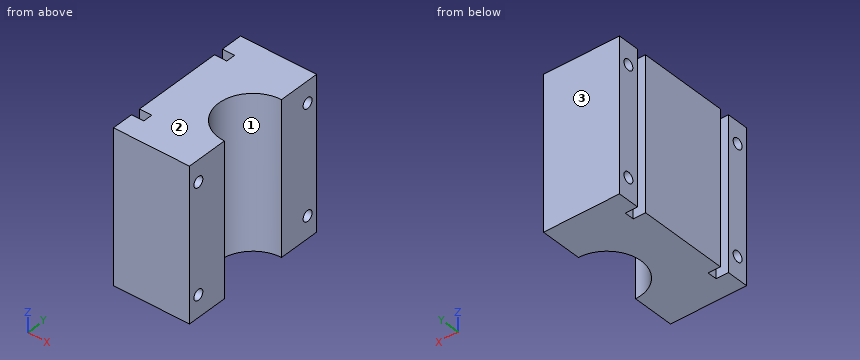
from build123d import *

# Parameters (mm, degrees)
F1_DEPTH = 50.8
F2_DEPTH = 50.8
F4_D     = 7.112


with BuildPart() as f1:
    # F0 (on Top) → F1 (new body)
    with BuildSketch(Plane.XY):
        with BuildLine():
            Line((-50.8, 0), (-22.86, 0))
            ThreePointArc((-22.86, 0), (-16.164461, 16.164461), (0, 22.86))
            Line((0, 22.86), (0, 50.8))
            Line((0, 50.8), (-50.8, 50.8))
            Line((-50.8, 50.8), (-50.8, 36.323187))
            Line((-50.8, 36.323187), (-42.600878, 36.323187))
            Line((-42.600878, 36.323187), (-42.600878, 29.973187))
            Line((-42.600878, 29.973187), (-50.8, 29.973187))
            Line((-50.8, 29.973187), (-50.8, 0))
        make_face()
        with BuildLine():
            ThreePointArc((0, -22.86), (-16.164461, -16.164461), (-22.86, 0))
            Line((-22.86, 0), (-50.8, 0))
            Line((-50.8, 0), (-50.8, -29.973187))
            Line((-50.8, -29.973187), (-42.600878, -29.973187))
            Line((-42.600878, -29.973187), (-42.600878, -36.323187))
            Line((-42.600878, -36.323187), (-50.8, -36.323187))
            Line((-50.8, -36.323187), (-50.8, -50.8))
            Line((-50.8, -50.8), (0, -50.8))
            Line((0, -50.8), (0, -22.86))
        make_face()
    extrude(amount=F1_DEPTH)

    # F1_face (on face) → F2 (join)
    with BuildSketch(Plane(origin=(-27.91822, 0, 50.8), x_dir=(1, 0, 0), z_dir=(0, 0, 1))):
        with BuildLine():
            Line((-14.682658, 36.323187), (-14.682658, 29.973187))
            Line((-14.682658, 29.973187), (-22.88178, 29.973187))
            Line((-22.88178, 29.973187), (-22.88178, -29.973187))
            Line((-22.88178, -29.973187), (-14.682658, -29.973187))
            Line((-14.682658, -29.973187), (-14.682658, -36.323187))
            Line((-14.682658, -36.323187), (-22.88178, -36.323187))
            Line((-22.88178, -36.323187), (-22.88178, -50.8))
            Line((-22.88178, -50.8), (27.91822, -50.8))
            Line((27.91822, -50.8), (27.91822, -22.86))
            ThreePointArc((27.91822, -22.86), (5.05822, 0), (27.91822, 22.86))
            Line((27.91822, 22.86), (27.91822, 50.8))
            Line((27.91822, 50.8), (-22.88178, 50.8))
            Line((-22.88178, 50.8), (-22.88178, 36.323187))
            Line((-22.88178, 36.323187), (-14.682658, 36.323187))
        make_face()
    extrude(amount=F2_DEPTH)

    # F4 (through all)
    with Locations(Plane(origin=(-50.8, 0, 0), x_dir=(0, -1, 0), z_dir=(-1, 0, 0))):
        with Locations((-43.662325, 87.244935), (43.662325, 87.244935), (43.662325, 14.645034), (-43.662325, 14.645034)):
            Hole(F4_D / 2)


solid = f1.part
Input: part model. Units: mm. Frame: model coordinates. Face numbers are marked on the shaded views. Coordinates: 2 decimals unless noted, no trailing zeros. Loops run counter-clockwise (first coordinate to the right, second up) from the corner with the lowest first, then second, coordinate; pieces in that order, holes last.
Q1. Cut plane B-B (z = 89). Output: boundary loops of the cut face in (x, y), then the cut area to 3 significant figures.
Q2. Contact query for flat-ended pins moving along their axis: pin 1 (11.5 mm diameter, centred on y = 43.66, z = 87.24, fed in from +X); pin 2 (3 mm diameter, centred on y = 34, z = 44, fed in from -X); pin 3 (5.5 mm diameter, centred on y = 43.66, z = 14.65, fed in from +X). Output: stop coordinate, or through.
Q3. Cut plane A-A (x = -20). Output: boundary loops of the cut face in (y, z).
Q4. Draft query along Y for the marked faces 1, 2 and 3. Return one class per face: +Y half, -Y half, draft (parallel to the pull), parting line (faces both ways), or undercut.
Q5. Material intervals for line 1 (Z direction, x = -23, y = -44) (3 decimals); line 2 (Z direction, x = -46, y = -45); line 3 (Y direction, x = -14, z = 87), sorted ascending.
Q6. Cut plane C-C (x = -46.5). Output: boundary loops of the cut face in (y, z), then the cut area to 3 significant figures.
Q7. Cut plane D-D (z = 41). Output: boundary loops of the cut face in (x, y).
Working result:
1. outline: (-50.8, -50.8) - (0, -50.8) - (0, -46.76) - (-50.8, -46.76) - close; (-50.8, -40.57) - (0, -40.57) - (0, -22.86) arc R22.86 cw to (0, 22.86) - (0, 40.57) - (-50.8, 40.57) - (-50.8, 36.32) - (-42.6, 36.32) - (-42.6, 29.97) - (-50.8, 29.97) - (-50.8, -29.97) - (-42.6, -29.97) - (-42.6, -36.32) - (-50.8, -36.32) - close; (-50.8, 46.76) - (0, 46.76) - (0, 50.8) - (-50.8, 50.8) - close
1. area: 3,610 mm2
2. pin 1: stops at x = 0
2. pin 2: stops at x = -42.6
2. pin 3: passes through
3. outline: (-50.8, 0) - (-11.07, 0) - (-11.07, 101.6) - (-50.8, 101.6) - close; (11.07, 0) - (50.8, 0) - (50.8, 101.6) - (11.07, 101.6) - close; hole circle Ø7.11 at (-43.66, 14.65); hole circle Ø7.11 at (-43.66, 87.24); hole circle Ø7.11 at (43.66, 14.65); hole circle Ø7.11 at (43.66, 87.24)
4. face 1: undercut
4. face 2: draft
4. face 3: +Y half
5. line 1: z = 0 to 11.105, 18.185 to 83.705, 90.785 to 101.6
5. line 2: z = 0 to 11.35, 17.94 to 83.95, 90.54 to 101.6
5. line 3: y = -50.8 to -47.21, -40.11 to -18.07, 18.07 to 40.11, 47.21 to 50.8
6. outline: (-50.8, 0) - (-36.32, 0) - (-36.32, 101.6) - (-50.8, 101.6) - close; (-29.97, 0) - (29.97, 0) - (29.97, 101.6) - (-29.97, 101.6) - close; (36.32, 0) - (50.8, 0) - (50.8, 101.6) - (36.32, 101.6) - close; hole circle Ø7.11 at (-43.66, 14.65); hole circle Ø7.11 at (-43.66, 87.24); hole circle Ø7.11 at (43.66, 14.65); hole circle Ø7.11 at (43.66, 87.24)
6. area: 8,870 mm2
7. outline: (-50.8, -50.8) - (0, -50.8) - (0, -22.86) arc R22.86 cw to (0, 22.86) - (0, 50.8) - (-50.8, 50.8) - (-50.8, 36.32) - (-42.6, 36.32) - (-42.6, 29.97) - (-50.8, 29.97) - (-50.8, -29.97) - (-42.6, -29.97) - (-42.6, -36.32) - (-50.8, -36.32) - close
